Can you work these out from the model? Positions are in its coordinate system, mm. Face numbers are marked on the shaded views. A direction names the side the tool comes from. Coordinates: 2 decimals unless noted, no trailing zeros. Order: outer loops, then holes, each group sorted by start corner. A loop starts at its lowest first (then second) coordinate and runs counter-clockwise, first axis right, second up. Notation, with made-up numbers: (14, 21.25) -> (47, 21.25) arc R23 ccw to (47, 56.25) -> close; hole circle Ø10 at (51.25, 67). An arc over 180 degrees is marked (long way). Answer in a Markdown table with one row per item.
```python
from build123d import *

# Parameters (mm, degrees)
SKETCH1_R               = 1.5
BOSS_EXTRUDE1_DEPTH     = 18
FILLET1_R               = 1.5
SKETCH2_R               = 1
SKETCH2_R_2             = 0.5
EXTRUDE_THIN1_DEPTH     = 2
EXTRUDE_THIN2_START     = -2
SKETCH2_2_R             = 1
SKETCH2_2_R_2           = 0.5
EXTRUDE_THIN2_DEPTH     = 2
CUT_EXTRUDE1_DEPTH      = 19.172781865
CUT_EXTRUDE1_DEPTH_BACK = 19.172781865
SKETCH3_R               = 0.5
SKETCH4_R               = 0.5
CUT_EXTRUDE2_DEPTH      = 3
SKETCH5_R               = 0.75
CUT_EXTRUDE3_DEPTH      = 17


with BuildPart() as part:
    # Sketch1 → Boss-Extrude1 (new body)
    with BuildSketch(Plane(origin=(0, 0, 0), x_dir=(1, 0, 0), z_dir=(0, 1, 0))):
        with Locations(Location((0, 0, 0), (0, 0, 270))):
            Circle(SKETCH1_R)
    extrude(amount=BOSS_EXTRUDE1_DEPTH)

    # Fillet1
    fillet1_edges = [part.edges().sort_by_distance(p)[0] for p in [
        (0, 18, -1.5),
    ]]
    fillet(fillet1_edges, radius=FILLET1_R)

    # Sketch2 → Extrude-Thin1 (add)
    # profile 1 of 2: a face of its own
    with BuildSketch(Plane.XY):
        with Locations((0, 7)):
            Circle(SKETCH2_R)
        with Locations((0, 7)):
            Circle(SKETCH2_R_2, mode=Mode.SUBTRACT)
    # profile 2 of 2: a face of its own
    with BuildSketch(Plane.XY):
        with Locations((0, 10)):
            Circle(SKETCH2_R)
        with Locations((0, 10)):
            Circle(SKETCH2_R_2, mode=Mode.SUBTRACT)
    extrude(amount=EXTRUDE_THIN1_DEPTH)

    # Sketch2_2 → Extrude-Thin2 (add)
    with BuildSketch(Plane.XY.offset(EXTRUDE_THIN2_START)):
        with Locations((0, 7)):
            Circle(SKETCH2_2_R)
        with Locations((0, 7)):
            Circle(SKETCH2_2_R_2, mode=Mode.SUBTRACT)
    extrude(amount=EXTRUDE_THIN2_DEPTH)

    # Sketch3 → Cut-Extrude1 (cut, two sides: drawn at the far end of the back side and taken through both)
    with BuildSketch(Plane.XY.offset(-CUT_EXTRUDE1_DEPTH_BACK)):
        with Locations((0, 7)):
            Circle(SKETCH3_R)
    extrude(amount=CUT_EXTRUDE1_DEPTH + CUT_EXTRUDE1_DEPTH_BACK, mode=Mode.SUBTRACT)

    # Sketch4 → Cut-Extrude2 (cut, symmetric)
    with BuildSketch(Plane(origin=(0, 0, 0), x_dir=(0.7071067811865477, 0, 0.7071067811865475), z_dir=(-0.7071067811865475, 0, 0.7071067811865477))):
        with Locations((0, 15)):
            Circle(SKETCH4_R)
    extrude(amount=CUT_EXTRUDE2_DEPTH, both=True, mode=Mode.SUBTRACT)

    # Sketch5 → Cut-Extrude3 (cut)
    with BuildSketch(Plane.XZ):
        with Locations(Location((0, 0, 0), (0, 0, 270))):
            Circle(SKETCH5_R)
    extrude(amount=-CUT_EXTRUDE3_DEPTH, mode=Mode.SUBTRACT)


solid = part.part
```
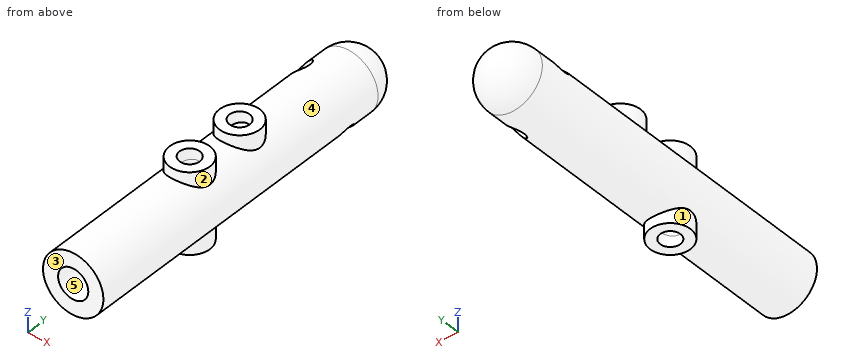
(1) Suppose I cut it at A-A (y = 7). Please give me the cut outline in (x, z).
Response values:
| item | result |
|---|---|
| outline | (-1, -2) -> (-0.5, -2) -> (-0.5, -0.56) arc R0.75 cw to (-0.5, 0.56) -> (-0.5, 2) -> (-1, 2) -> (-1, 1.12) arc R1.5 ccw to (-1, -1.12) -> close; (0.5, -2) -> (1, -2) -> (1, -1.12) arc R1.5 ccw to (1, 1.12) -> (1, 2) -> (0.5, 2) -> (0.5, 0.56) arc R0.75 cw to (0.5, -0.56) -> close |
(2) Suppose I cut it at B-B (y = 11.5). Please give me the cut outline in (x, z).
Response values:
| item | result |
|---|---|
| outline | circle Ø3 at (0, 0); hole circle Ø1.5 at (0, 0) |
(3) I need wall thicknesses on line 1 (Y direction, x = 0, z = 1.8); line 2 (X direction, y = 10.75, z = 0); line 3 (X direction, y = 10, z = 1.85). Which ranges of each line are inside material? Lowest first, please. Write a range as [from, to].
Response values:
| item | result |
|---|---|
| line 1 | [6, 6.5], [7.5, 8], [9, 9.5], [10.5, 11] |
| line 2 | [-1.5, -0.75], [0.75, 1.5] |
| line 3 | [-1, -0.5], [0.5, 1] |
(4) On a 3-axis mill with a long thin cutter (end or side, diameter ignored), from which of +Z, -Z, +X, -X, +Y, -Y can I reach the whole of each face in a straight line? I mean the marked faces 1 and 2. Say none if no direction works.
Response values:
| item | result |
|---|---|
| face 1 | -Z |
| face 2 | +Z |
(5) We'd pull the mould along X, two halves only. Please class the marked faces 3, 4 and 5: +X half, -X half, draft (parallel to the pull), parting line (faces both ways), or undercut.
Response values:
| item | result |
|---|---|
| face 3 | draft |
| face 4 | parting line |
| face 5 | undercut |
